Can you work these out from the drawing? Everything is in mm from the part's minimum corner. A direction names the side the tool comes from. Coordinates: 2 decimals unless noted, no trailing zeros. Order: outer loops, then holes, each group sorted by start corner. A loop starts at its lowest first (then second) coordinate and runs counter-clockwise, first axis right, second up. Notation, with made-up numbers: (11, 87.25) - (59, 87.25) arc R19 cw to (59, 117.25) - close; hole circle Ø2 at (7, -29). An arc over 180 degrees is marked (long way). Use a Markdown table: item, result. Add a question column.
(1) On a 3-axis mill with a long thin cutter (end or side, diameter ignored), from which of +Z, -Z, +X, -X, +Y, -Y can I reach the whole of each face in a straight line? I mean the marked faces 1, 2 and 3. Say none if no direction works.
(2) I want a section at A-A (y = 6). List the corners of the cut face in (x, z) for me (3 decimals).
(3) For pin 1 Ø3 at (x, y) = (4.5, 5) entering from -Z; pin 2 Ø1.5 at (y, z) = (2, 4.5) entering from -X, each with a flat end and sliding along its axis, tell me the tip position at first contact or that it passes through.
(4) I want a section at C-C (z = 16.75). List the corners of the cut face in (x, y) for me (3 decimals).
(5) If I drill on L1, parallel to Y at x = 6, z = 13.75 (3 decimals); L2, parallel to Z at x = 11.5, y = 5; L3, parallel to Y at x = 5.5, z = 6.5, over which ranges is the centre line in solid material (lowest first)? Write a range as [from, to].
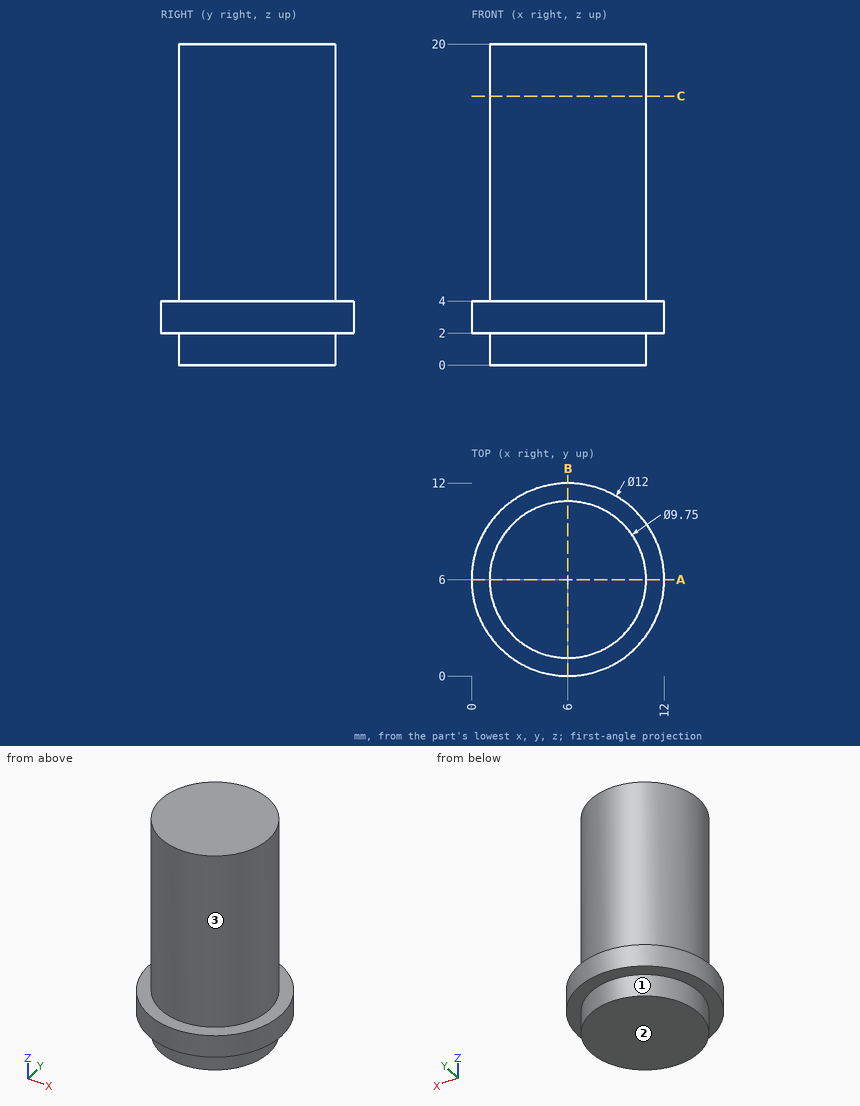
Answers follow:
| question | item | result |
|---|---|---|
| 1 | face 1 | -Z |
| 1 | face 2 | -Z, +X, -X, +Y, -Y |
| 1 | face 3 | +Z |
| 2 | outline | (0, 2) - (1.125, 2) - (1.125, 0) - (10.875, 0) - (10.875, 2) - (12, 2) - (12, 4) - (10.875, 4) - (10.875, 20) - (1.125, 20) - (1.125, 4) - (0, 4) - close |
| 3 | pin 1 | stops at z = 0 |
| 3 | pin 2 | stops at x = 1.08 |
| 4 | outline | circle Ø9.75 at (6, 6) |
| 5 | L1 | y = [1.125, 10.875] |
| 5 | L2 | z = [2, 4] |
| 5 | L3 | y = [1.15, 10.85] |
